Here's the drawing with two shaded views (mm, measured from the low corner). I have some questions. Coordinates: 2 decimals unless noted, no trailing zeros. Order: outer loops, then holes, each group sorted by start corner. A loop starts at its lowest first (then second) coordinate and runs counter-clockwise, first axis right, second up. Notation, with made-up numbers: (49.25, 19) -> (65.25, 19) arc R18 cw to (65.25, 53) -> close; hole circle Ø10 at (89, 75.5). An arc over 180 degrees is marked (long way). Answer as a JSON object with one key per item and string values. Group by question number.
(1) For pin 1 (2 mm diameter, centred on y = 23, z = 3, fed in from -X); pin 2 (3 mm diameter, centred on y = 21.5, z = 4.5, fed in from +X), each with a flat end and sliding along its axis, tell me the tip position at first contact or that it passes through.
(2) I want a section at C-C, the plane x = 18. List the corners of the cut face in (y, z) for me, plus the area to 3 significant figures.
(3) I want a section at A-A, the plane x = 25. List the corners of the cut face in (y, z) for me.
(4) I want a section at B-B, the plane y = 17. List the corners of the cut face in (x, z) for me (1 decimal), plus the area to 3 significant figures.
(5) I need wall thicknesses on line 1 (Y direction, x = 25, z = 3.8); line 2 (X direction, y = 12, z = 0.9) (1 decimal); line 3 (X direction, y = 17, z = 1.35) (1 decimal). Which ranges of each line are inside material? Lowest first, please.
(6) If we mould it in two halves opening along Y, with no side actions, what happens to the marked faces 1, 2, 3 and 4? For each: pulls with the +Y half, pulls with the -Y half, needs draft (parallel to the pull), parting line crosses it, or undercut.
(7) I want a section at D-D, the plane z = 2.4. List the corners of the cut face in (x, y) for me, plus the area to 3 significant figures.
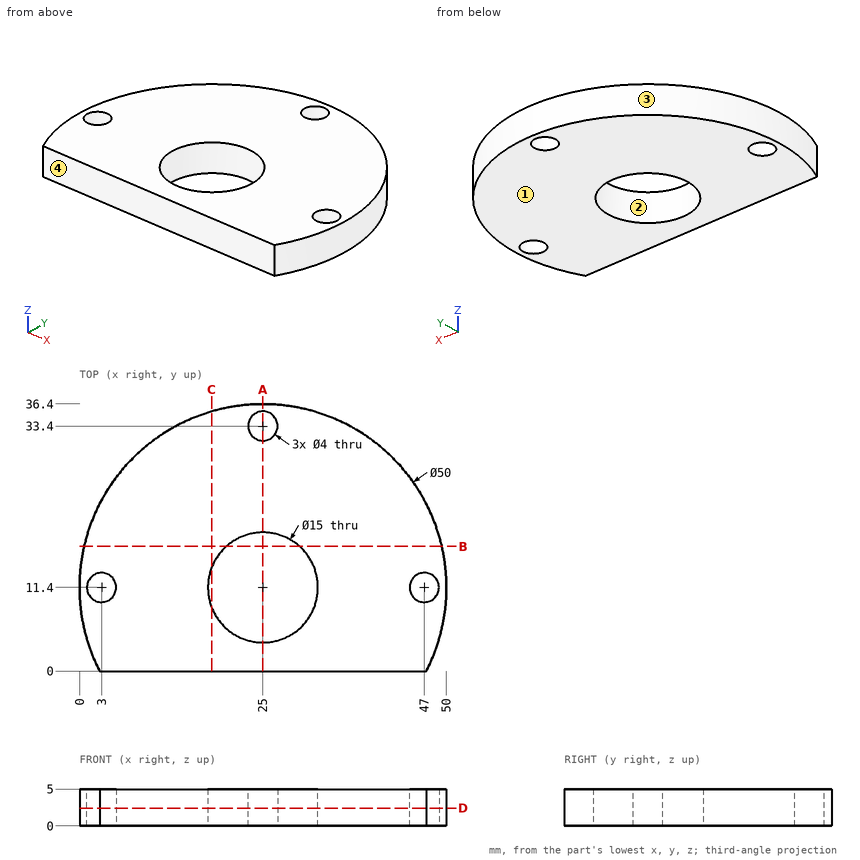
Computed values:
{
 "1": {"pin 1": "stops at x = 2.36", "pin 2": "stops at x = 48.47"},
 "2": {"outline": "(0, 0) -> (8.71, 0) -> (8.71, 5) -> (0, 5) -> close; (14.09, 0) -> (35.4, 0) -> (35.4, 5) -> (14.09, 5) -> close", "area": "150 mm2"},
 "3": {"outline": "(0, 0) -> (3.9, 0) -> (3.9, 5) -> (0, 5) -> close; (18.9, 0) -> (31.4, 0) -> (31.4, 5) -> (18.9, 5) -> close; (35.4, 0) -> (36.4, 0) -> (36.4, 5) -> (35.4, 5) -> close"},
 "4": {"outline": "(0.6, 0) -> (20, 0) -> (20, 5) -> (0.6, 5) -> close; (30, 0) -> (49.4, 0) -> (49.4, 5) -> (30, 5) -> close", "area": "194 mm2"},
 "5": {"line 1": "y = 0 to 3.9, 18.9 to 31.4, 35.4 to 36.4", "line 2": "x = 0 to 1.1, 4.9 to 17.5, 32.5 to 45.1, 48.9 to 50", "line 3": "x = 0.6 to 20, 30 to 49.4"},
 "6": {"face 1": "needs draft", "face 2": "undercut", "face 3": "parting line crosses it", "face 4": "pulls with the -Y half"},
 "7": {"outline": "(2.75, 0) -> (47.25, 0) arc R25 ccw (long way) to start; hole circle Ø4 at (3, 11.4); hole circle Ø15 at (25, 11.4); hole circle Ø4 at (25, 33.4); hole circle Ø4 at (47, 11.4)", "area": "1,320 mm2"}
}
